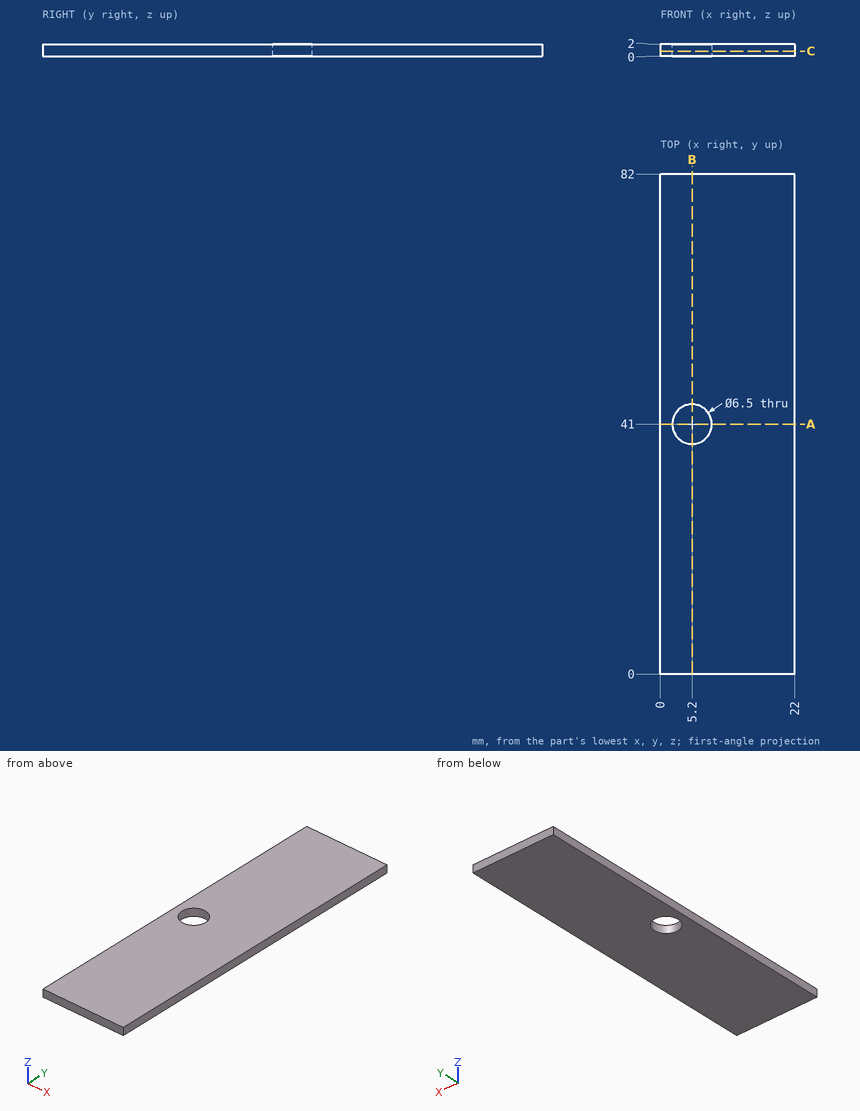
Print and shaded views of the part. All mm, measured from the part's lowest x, y and z. Round coordinates to 2 decimals unless told otherwise and drop trailing zeros. Order: outer loops, then holes, each group sorted by start corner. A loop starts at its lowest first (then second) coordinate and runs counter-clockwise, first axis right, second up. Notation, with made-up numbers: (-30, 42.5) - (26, 42.5) arc R22 ccw to (26, 77.5) - close; hole circle Ø4 at (10.25, 76.5). An arc over 180 degrees is marked (long way). Use a Markdown table: item, result.
1) Wall check: L1, parallel to Y at x = 5.2, z = 0.6; L2, parallel to Y at x = 7, z = 1.1; L3, parallel to X at y = 40, z = 1.8. Give the ranges that are in metal, low to high.
Recorded:
| item | result |
|---|---|
| L1 | y = 0 to 37.75, 44.25 to 82 |
| L2 | y = 0 to 38.29, 43.71 to 82 |
| L3 | x = 0 to 2.11, 8.29 to 22 |
2) Saw through at B-B on x = 5.2. Write the cut outline in (y, z), and give its area (3 significant figures).
Recorded:
| item | result |
|---|---|
| outline | (0, 0) - (37.75, 0) - (37.75, 2) - (0, 2) - close; (44.25, 0) - (82, 0) - (82, 2) - (44.25, 2) - close |
| area | 151 mm² |
3) Saw through at A-A on y = 41. Write the cut outline in (x, z).
Recorded:
| item | result |
|---|---|
| outline | (0, 0) - (1.95, 0) - (1.95, 2) - (0, 2) - close; (8.45, 0) - (22, 0) - (22, 2) - (8.45, 2) - close |
4) Saw through at C-C on z = 0.85. Write the cut outline in (x, y), and give its area (3 significant figures).
Recorded:
| item | result |
|---|---|
| outline | (0, 0) - (22, 0) - (22, 82) - (0, 82) - close; hole circle Ø6.5 at (5.2, 41) |
| area | 1,770 mm² |
